Geometry: final body of the model. Coordinates: model frame, mm. A direction names the side the tool comes from. Give positions to 0.01 mm unless a question says otherwise; leave off trailing zeros. Write each loop counter-clockwise with the first axis right and the second up, starting at its lowest first coordinate (ties: lowest second). Pieces come first, ordered by that corner, then holes.
Autodesk Inventor part; units mm, degrees
ref_plane "YZ Plane" through (0, 0, 0) normal (1, 0, 0) x (0, 1, 0)
ref_plane "XZ Plane" through (0, 0, 0) normal (0, 1, 0) x (-1, 0, 0)
ref_plane "XY Plane" through (0, 0, 0) normal (0, 0, 1) x (1, 0, 0)
sketch "Sketch_2" plane through (0, 0, 0) normal (0, 0, 1) x (1, 0, 0)
  line L0 (8, 0) -> (0, 0)
  line L1 (0, 2.4) -> (0.2, 2.2)
  line L2 (0.2, 2.2) -> (0.2, 2)
  line L3 (0.2, 2) -> (6.27, 2)
  line L4 (6.27, 2) -> (6.5, 2.05)
  line L5 (6.5, 2.05) -> (7.8, 2.05)
  line L6 (7.8, 2.05) -> (7.8, 2.25)
  line L7 (7.8, 2.25) -> (8, 2.45)
  line L8 (8, 2.45) -> (8, 5.6)
  line L9 (8, 5.6) -> (7.8, 5.8)
  line L10 (7.8, 5.8) -> (7.8, 6)
  line L11 (7.8, 6) -> (3.5, 6)
  arc A0 (3, 6.5) -> (3.5, 6) centre (3.5, 6.5) ccw
  line L12 (3, 6.5) -> (3, 19.175)
  line L13 (3, 19.175) -> (2.7664, 20.5)
  line L14 (2.7664, 20.5) -> (0.2336, 20.5)
  line L15 (0.2336, 20.5) -> (0, 19.175)
  line L16 (0, 19.175) -> (0, 2.4)
revolve "Revolution1" add sketch "Sketch_2" angle 360 about axis through (8, 0, 0) along (1, 0, 0)
sketch "Sketch_3" plane through (0, 0, 0) normal (0, 0, 1) x (1, 0, 0)
  line L0 (0.75, 0) -> (0, 0)
  line L1 (-2, 18.25) -> (-2, 6)
  line L2 (-2, 6) -> (0, 6)
  line L3 (0, 6) -> (0.75, 6.75)
  line L4 (0.75, 6.75) -> (0.75, 17.817)
  line L5 (0.75, 17.817) -> (0, 18.25)
  line L6 (0, 18.25) -> (-2, 18.25)
revolve "Revolution2" cut sketch "Sketch_3" angle 360 about axis through (0.75, 0, 0) along (1, 0, 0)
sketch "Sketch_4" plane through (0, 0, 0) normal (0, 0, 1) x (1, 0, 0)
  line L0 (3, 0) -> (2.25, 0)
  line L1 (2.25, 17.75) -> (2.25, 6.5)
  arc A0 (2.25, 6.5) -> (2.75, 6) centre (2.75, 6.5) ccw
  line L2 (2.75, 6) -> (5, 6)
  line L3 (5, 6) -> (5, 18.25)
  line L4 (5, 18.25) -> (2.75, 18.25)
  arc A1 (2.75, 18.25) -> (2.25, 17.75) centre (2.75, 17.75) ccw
revolve "Revolution3" cut sketch "Sketch_4" angle 360 about axis through (3, 0, 0) along (1, 0, 0)
properties part number "焼結ギア" material "鋼、高強度、低合金"
Item 1: Pull-direction query (Z, two-part tool) for faces 1 (the face through (0.75, 8, 0)), 2 (the face through (1.482, -4.444, 20.013)), 3 (the face through (8, 2.4, -1.2)), 4 (the face through (3, 0, -2)); classes: +Z half, -Z half, draft (parallel to the pull), parting line (faces both ways), or undercut.
Found:
face 1: undercut
face 2: parting line
face 3: draft
face 4: undercut
Item 2: Section A-A, the plane x = 7. Return the cut outline in (y, z).
Found:
outline: circle Ø12 at (0, 0); hole circle Ø4.1 at (0, 0)
Item 3: Pin query (flat end, axial travel): pin 1 Ø4 at (x, y) = (4.5, -12.5) entering from -Z; pin 2 Ø1 at (x, y) = (2.5, -2.5) entering from +Z; pin 3 Ø5 at (y, z) = (-1, -8.5) entering from -X. Return the tip coordinate at first contact, or that it passes through.
Found:
pin 1: stops at z = -16.97
pin 2: stops at z = 20.4
pin 3: stops at x = 0.06
Item 4: Line query: L1, parallel to Z at x = 6.95, y = 0; L2, parallel to Z at x = 2.5, y = 0; L3, parallel to X at y = 13, z = 12. Output: solid intervals per line, ascending.
Found:
L1: z = -6 to -2.05, 2.05 to 6
L2: z = -20.5 to -18.18, -6.07 to -2, 2 to 6.07, 18.18 to 20.5
L3: x = 0.75 to 2.25
Item 5: Section B-B, the plane x = 1.25. Return the cut outline in (y, z), plus the area to 3 significant figures.
Found:
outline: circle Ø41 at (0, 0); hole circle Ø4 at (0, 0)
area: 1,310 mm2
Item 6: Reachability of faces 5 (the face through (0, 3, 0)), 6 (the face through (5, -6, 0)) from +Z, -Z, +X, -X, +Y, -Y: full face, straight path, thin tool, end or side. Return the list, or none.
Found:
face 5: +Z, -Z, -X, +Y, -Y
face 6: +X
